Check sheet for the drawn part. Datum: minimum x, y, z corner. Units: mm. A direction names the side the tool comes from. Give positions to 0.01 mm unless a question says otherwise; leave off trailing zeros. Write each loop counter-clockwise with the first axis right and the second up, starting at its lowest first coordinate (ties: lowest second). Pieces come first, ordered by that corner, then holes. Notation, with made-up numbers: M -6.5,-26.5 L 38.5,-26.5 A11 ccw 38.5,-22.5 Z; hole C 0,21.25 d4. An arc over 180 degrees is marked long. Write item = value, one per line. Start each with the question number.
1) Gauge pin test, flat ends, axial feed: pin 1 (0.6 mm diameter, centred on x = 27.5, z = 23, fed in from +Y); pin 2 (2 mm diameter, centred on y = 28, z = 8.5, fed in from -X); pin 3 (2.5 mm diameter, centred on x = 52.5, z = 12, fed in from +Y). Record the tip position at first contact, or that the pin passes through.
2) Sectioned sample at B-B, the plane x = 52.5. Record the cut outline in (y, z), then the cut area to 4 significant figures.
3) Sectioned sample at C-C, the plane y = 22. Record the cut outline in (x, z), then the cut area to 3 significant figures.
4) Sectioned sample at D-D, the plane z = 12. Record the cut outline in (x, y), then the cut area to 3 significant figures.
5) Draft check along Z on the marked faces 3, 4 and 5. Enter one of: pulls with the +Z half, pulls with the -Z half, needs draft (parallel to the pull), parting line crosses it, or undercut.
6) Set-up check for the marked faces 1 and 2: record each of +Z, -Z, +X, -X, +Y, -Y from which the full face is reachable in a straight line by a thin tool's end or side.
7) Sectioned sample at A-A, the plane y = 32. Record the cut outline in (x, z).
8) Scan lines: L1, parallel to X at y = 39, z = 12; L2, parallel to Y at x = 29.5, z = 8; L3, parallel to X at y = 26.5, z = 4. Record each from-to range of solid material in increasing order.
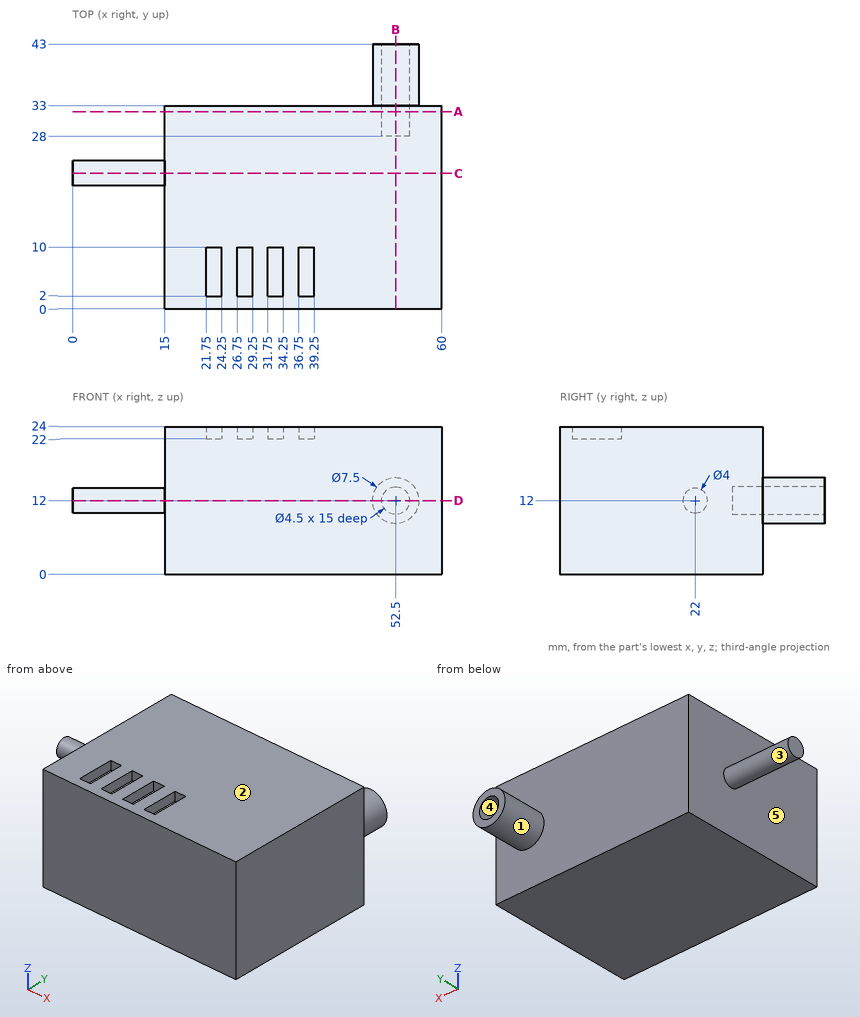
Data:
q1.pin_1 = 33
q1.pin_2 = 15
q1.pin_3 = 28
q2.outline = M 0,0 L 33,0 L 33,8.25 L 43,8.25 L 43,9.75 L 28,9.75 L 28,14.25 L 43,14.25 L 43,15.75 L 33,15.75 L 33,24 L 0,24 Z
q2.area = 799.5 mm2
q3.outline = M 0,10 L 15,10 L 15,0 L 60,0 L 60,24 L 15,24 L 15,14 L 0,14 Z
q3.area = 1,140 mm2
q4.outline = M 0,20 L 15,20 L 15,0 L 60,0 L 60,33 L 56.25,33 L 56.25,43 L 54.75,43 L 54.75,28 L 50.25,28 L 50.25,43 L 48.75,43 L 48.75,33 L 15,33 L 15,24 L 0,24 Z
q4.area = 1,550 mm2
q5.face_3 = parting line crosses it
q5.face_4 = undercut
q5.face_5 = needs draft
q6.face_1 = +Y
q6.face_2 = +Z, +X, -X, +Y, -Y
q7.outline = M 15,0 L 60,0 L 60,24 L 15,24 Z; hole C 52.5,12 d4.5
q8.L1 = 48.75 to 50.25, 54.75 to 56.25
q8.L2 = 0 to 33
q8.L3 = 15 to 60
